The listing builds one solid part. Answer for the finished solid, in the listing's coordinates (mm). Face numbers are marked on the shaded views. Coordinates: 2 decimals unless noted, no trailing zeros. Write each loop counter-clockwise with the first axis right and the second up, starting at its lowest first coordinate (ties: lowest second). Pieces come first, ordered by that corner, then holes.
from build123d import *

# Parameters (mm, degrees)
SKETCH1_W             = 2
SKETCH1_H             = 3
BOSS_EXTRUDE1_DEPTH   = 6
BOSS_EXTRUDE1_2_DEPTH = 6
BOSS_EXTRUDE1_3_DEPTH = 6
BOSS_EXTRUDE1_4_DEPTH = 6
BOSS_EXTRUDE1_5_DEPTH = 6
BOSS_EXTRUDE1_6_DEPTH = 6
BOSS_EXTRUDE1_7_DEPTH = 6
SKETCH2_W             = 80
SKETCH2_H             = 14
BOSS_EXTRUDE2_DEPTH   = 2
FILLET1_R             = 1
FILLET2_R             = 0.5


with BuildPart() as part:
    # Sketch1 → Boss-Extrude1 (new body)
    with BuildSketch(Plane(origin=(0, 0, 0), x_dir=(1, 0, 0), z_dir=(0, 1, 0))):
        with Locations((20, 10.5)):
            Rectangle(SKETCH1_W, SKETCH1_H)
    extrude(amount=BOSS_EXTRUDE1_DEPTH)



with BuildPart() as body_2:
    # Sketch1 → Boss-Extrude1 2 (new body)
    with BuildSketch(Plane(origin=(0, 0, 0), x_dir=(1, 0, 0), z_dir=(0, 1, 0))):
        with Locations((30, 3.5)):
            Rectangle(SKETCH1_W, SKETCH1_H)
    extrude(amount=BOSS_EXTRUDE1_2_DEPTH)


with BuildPart() as body_3:
    # Sketch1 → Boss-Extrude1 3 (new body)
    with BuildSketch(Plane(origin=(0, 0, 0), x_dir=(1, 0, 0), z_dir=(0, 1, 0))):
        with Locations((40, 10.5)):
            Rectangle(SKETCH1_W, SKETCH1_H)
    extrude(amount=BOSS_EXTRUDE1_3_DEPTH)


with BuildPart() as body_4:
    # Sketch1 → Boss-Extrude1 4 (new body)
    with BuildSketch(Plane(origin=(0, 0, 0), x_dir=(1, 0, 0), z_dir=(0, 1, 0))):
        with Locations((50, 3.5)):
            Rectangle(SKETCH1_W, SKETCH1_H)
    extrude(amount=BOSS_EXTRUDE1_4_DEPTH)


with BuildPart() as body_5:
    # Sketch1 → Boss-Extrude1 5 (new body)
    with BuildSketch(Plane(origin=(0, 0, 0), x_dir=(1, 0, 0), z_dir=(0, 1, 0))):
        with Locations((60, 10.5)):
            Rectangle(SKETCH1_W, SKETCH1_H)
    extrude(amount=BOSS_EXTRUDE1_5_DEPTH)


with BuildPart() as body_6:
    # Sketch1 → Boss-Extrude1 6 (new body)
    with BuildSketch(Plane(origin=(0, 0, 0), x_dir=(1, 0, 0), z_dir=(0, 1, 0))):
        with Locations((70, 3.5)):
            Rectangle(SKETCH1_W, SKETCH1_H)
    extrude(amount=BOSS_EXTRUDE1_6_DEPTH)


with BuildPart() as body_7:
    # Sketch1 → Boss-Extrude1 7 (new body)
    with BuildSketch(Plane(origin=(0, 0, 0), x_dir=(1, 0, 0), z_dir=(0, 1, 0))):
        with Locations((10, 3.5)):
            Rectangle(SKETCH1_W, SKETCH1_H)
    extrude(amount=BOSS_EXTRUDE1_7_DEPTH)


with BuildPart() as part_1:
    add(part.part)

    add(body_2.part)  # Boss-Extrude2 merges body 2

    add(body_3.part)  # Boss-Extrude2 merges body 3

    add(body_4.part)  # Boss-Extrude2 merges body 4

    add(body_5.part)  # Boss-Extrude2 merges body 5

    add(body_6.part)  # Boss-Extrude2 merges body 6

    add(body_7.part)  # Boss-Extrude2 merges body 7
    # Sketch2 → Boss-Extrude2 (add)
    with BuildSketch(Plane.XZ):
        with Locations((40, -7)):
            Rectangle(SKETCH2_W, SKETCH2_H)
    extrude(amount=BOSS_EXTRUDE2_DEPTH)

    # Fillet1
    fillet1_edges = [part_1.edges().sort_by_distance(p)[0] for p in [
        (0, -2, -7),
        (40, -2, -14),
        (80, -2, -7),
        (40, -2, 0),
    ]]
    fillet(fillet1_edges, radius=FILLET1_R)

    # Fillet2
    fillet2_edges = [part_1.edges().sort_by_distance(p)[0] for p in [
        (20, 6, -9),
        (51, 6, -3.5),
        (50, 6, -5),
        (49, 6, -3.5),
        (50, 6, -2),
        (61, 6, -10.5),
        (60, 6, -12),
        (59, 6, -10.5),
        (60, 6, -9),
        (71, 6, -3.5),
        (70, 6, -5),
        (69, 6, -3.5),
        (70, 6, -2),
        (10, 6, -5),
        (11, 6, -3.5),
        (9, 6, -3.5),
        (10, 6, -2),
        (21, 6, -10.5),
        (20, 6, -12),
        (19, 6, -10.5),
        (31, 6, -3.5),
        (30, 6, -5),
        (29, 6, -3.5),
        (30, 6, -2),
        (41, 6, -10.5),
        (40, 6, -12),
        (39, 6, -10.5),
        (40, 6, -9),
    ]]
    fillet(fillet2_edges, radius=FILLET2_R)


solid = part_1.part
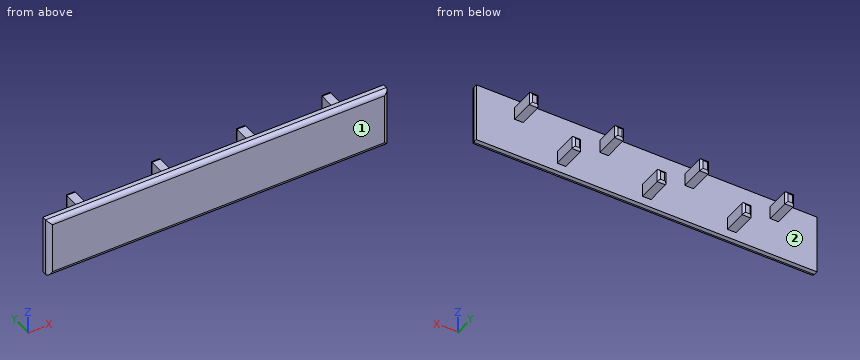
1. Flat-ended cylindrical pins translate along their axes: P1, Ø1.6, axis at x = 20.5, y = 4, coming from the -Z side; P2, Ø1.5, axis at y = 2, z = -10, coming from the -X side; P3, Ø1.5, axis at y = 2, z = -3.5, coming from the -X side. Find the tip coordinate at first contact, or state that the pin passes through.
Results found:
P1: stops at z = -12
P2: stops at x = 19
P3: stops at x = 9
2. Section C-C on x = 23 is taken. Give the vertices of the cut face in (y, z).
Results found:
outline: (-2, -13) arc R1 ccw to (-1, -14) - (0, -14) - (0, 0) - (-1, 0) arc R1 ccw to (-2, -1) - close
3. For a pull along X with two mould halves and no side action, classify the marked faces 1 and 2 as pulls with the +X half, pulls with the -X half, needs draft (parallel to the pull), parting line crosses it, or undercut.
Results found:
face 1: needs draft
face 2: undercut
4. Section D-D on z = -7 is taken. Give the vertices of the cut face in (x, y).
Results found:
outline: (0, -1) arc R1 ccw to (1, -2) - (79, -2) arc R1 ccw to (80, -1) - (80, 0) - (0, 0) - close
5. Section A-A on y = 4.5 is taken. Give the vertices of the cut face in (x, z).
Results found:
outline: (9, -5) - (11, -5) - (11, -2) - (9, -2) - close; (19, -12) - (21, -12) - (21, -9) - (19, -9) - close; (29, -5) - (31, -5) - (31, -2) - (29, -2) - close; (39, -12) - (41, -12) - (41, -9) - (39, -9) - close; (49, -5) - (51, -5) - (51, -2) - (49, -2) - close; (59, -12) - (61, -12) - (61, -9) - (59, -9) - close; (69, -5) - (71, -5) - (71, -2) - (69, -2) - close
6. Find the intervals of material crossed by L1, parallel to X at y = 1, z = -2.75; L2, parallel to X at y = 1.5, z = -9.75; L3, parallel to X at y = 5.75, z = -4.5, in increasing order.
Results found:
L1: x = 9 to 11, 29 to 31, 49 to 51, 69 to 71
L2: x = 19 to 21, 39 to 41, 59 to 61
L3: x = 9.07 to 10.93, 29.07 to 30.93, 49.07 to 50.93, 69.07 to 70.93
